Could you check a few things on this model? Use its own coordinates, in mm. Coordinates: 2 decimals unless noted, no trailing zeros. Loops run counter-clockwise (first coordinate to the right, second up) from the corner with the lowest first, then second, coordinate; pieces in that order, holes last.
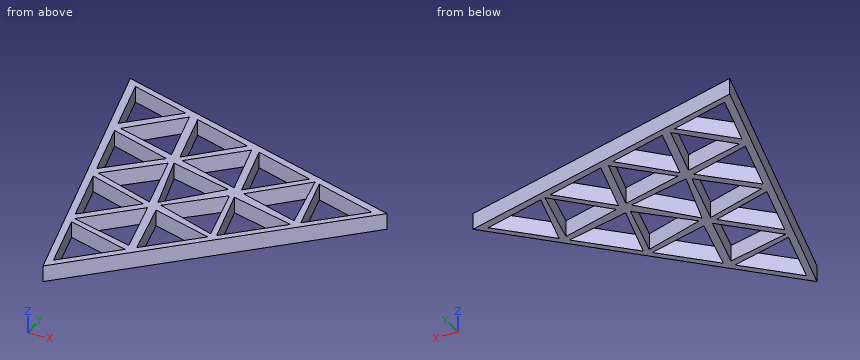
from build123d import *

# Parameters (mm, degrees)
RESSALTO_EXTRUS_O1_DEPTH = 10


with BuildPart() as part:
    # Esboço1 → Ressalto-extrusão1 (new body)
    with BuildSketch(Plane.XY):
        Polygon((-126.238515457, 94.285443038), (-80.275914767, -91.055638665), (58.278900907, 41.674126668), align=None)
        Polygon((-120.027353202, 88.571173763), (-111.121083647, 52.102898426), (-83.875189284, 78.078561997), align=None, mode=Mode.SUBTRACT)
        Polygon((-78.039896355, -83.353797468), (-49.163405973, -55.823557892), (-87.332121667, -45.305158912), align=None, mode=Mode.SUBTRACT)
        Polygon((-107.605028691, 48.322842348), (-80.275914767, 75.651956272), (-71.247120871, 38.363415453), align=None, mode=Mode.SUBTRACT)
        Polygon((-75.120650095, 75.537691107), (-66.114464824, 38.342522964), (-39.312161848, 65.14482594), align=None, mode=Mode.SUBTRACT)
        Polygon((-109.376188137, 44.95811918), (-71.828734099, 33.664499425), (-100.202444106, 7.394622908), align=None, mode=Mode.SUBTRACT)
        Polygon((-30.847981962, 62.688227391), (-21.624691556, 25.38847633), (5.623637916, 52.102898426), align=None, mode=Mode.SUBTRACT)
        Polygon((-68.847376217, 30.186248562), (-97.418722592, 3.850920598), (-59.73906137, -8.361685457), align=None, mode=Mode.SUBTRACT)
        Polygon((-63.381553432, 35.900517837), (-35.418223954, 62.688227391), (-26.168285688, 25.38847633), align=None, mode=Mode.SUBTRACT)
        Polygon((-18.862754173, 22.543823465), (9.555234971, 50.961812609), (17.612002379, 11.801208285), align=None, mode=Mode.SUBTRACT)
        Polygon((12.511037677, 50.103936153), (21.768265533, 11.801208285), (50.407351595, 39.105111568), align=None, mode=Mode.SUBTRACT)
        Polygon((-98.396531864, 0), (-61.642428, -11.552761795), (-89.166567856, -37.793698777), align=None, mode=Mode.SUBTRACT)
        Polygon((-66.114464824, 31.676927503), (-55.431265745, -6.583831991), (-28.102151821, 22.543823465), align=None, mode=Mode.SUBTRACT)
        Polygon((-52.698354353, -8.361685457), (-24.623900958, 17.26703107), (-15.813359557, -20.575447504), align=None, mode=Mode.SUBTRACT)
        Polygon((-44.457092929, -51.33665786), (-52.698354353, -13.788780207), (-15.813359557, -24.02832393), align=None, mode=Mode.SUBTRACT)
        Polygon((-21.624691556, 17.26703107), (-12.191634703, -20.575447504), (17.612002379, 7.838714269), align=None, mode=Mode.SUBTRACT)
        Polygon((-57.915730647, -13.788780207), (-49.163405973, -51.33665786), (-87.332121667, -41.863233602), align=None, mode=Mode.SUBTRACT)
    extrude(amount=RESSALTO_EXTRUS_O1_DEPTH)


solid = part.part
(1) Imagine slicing it at B-B, the plane y = -72. Write out the boundary of the cut face in (x, z).
Answers:
outline: (-85, 0) - (-80.81, 0) - (-80.81, 10) - (-85, 10) - close; (-66.13, 0) - (-60.38, 0) - (-60.38, 10) - (-66.13, 10) - close
(2) Imagine slicing it at C-C, the plane z = 7.5. State how many separate pieces and enclosed holes the cut face has, and give its area (3 significant figures).
Answers:
separate pieces: 1
enclosed holes: 16
area: 5,410 mm2
(3) I need wall thicknesses on probe 1 along Y at (x, z) = (-3, 4.75); probe 2 along Y at (x, z) = (-5, 8.5); probe 3 along X at (y, z) = (-63, 2). Which ranges of each line are inside material? Lowest first, please.
Answers:
probe 1: y = -17.03 to -11.81, 12.79 to 17.87, 38.41 to 43.65, 54.61 to 59.15
probe 2: y = -18.94 to -13.72, 13.27 to 18.46, 36.41 to 41.69, 55.19 to 59.72
probe 3: x = -87.23 to -83.01, -56.69 to -50.99
(4) For pin 1 (3 mm diameter, centred on y = 55, z = 7, fed in from -X); pin 2 (3 mm diameter, centred on y = -36.5, z = 5, fed in from +X); pin 3 (6 mm diameter, centred on y = -17, z = 3, fed in from -X); pin 4 (8 mm diameter, centred on x = -67.5, y = 4.5, fed in from -Z), each with a flat end and sliding along its axis, tell me the tip position at first contact or that it passes through.
Answers:
pin 1: stops at x = -116.87
pin 2: stops at x = -21.76
pin 3: stops at x = -99.38
pin 4: passes through
(5) Imagine slicing it at A-A, the plane x = 39.5. Write out the boundary of the cut face in (y, z).
Answers:
outline: (23.68, 0) - (28.71, 0) - (28.71, 10) - (23.68, 10) - close; (42.27, 0) - (47.03, 0) - (47.03, 10) - (42.27, 10) - close
